The model under review builds one solid part; all positions refer to its coordinate system, in mm. A direction names the side the tool comes from. Give positions to 0.01 mm unless a question says otherwise; leave off trailing zeros. Order: outer loops, then holes, each group sorted by start corner. A loop starts at its lowest first (then second) coordinate and runs counter-clockwise, first axis right, second up. Notation, with made-up numbers: (65.5, -12.5) -> (116.5, -12.5) arc R15 ccw to (116.5, -3.5) -> close; hole circle Ø4 at (32, -22.5). An arc over 180 degrees is marked (long way). Use one line per item in the form item = value.
```python
from build123d import *

# Parameters (mm, degrees)
SKETCH_1_W                   = 310
SKETCH_1_H                   = 120
EXTRUDE_1_DEPTH              = 15
SKETCH_2_W                   = 260
SKETCH_2_H                   = 60
CUT_EXTRUDE_1_DEPTH          = 333.753662639
HOLE_WIZARD_M5_1_D           = 5.8
HOLE_WIZARD_M5_1_CBORE_D     = 10
HOLE_WIZARD_M5_1_CBORE_DEPTH = 5
SKETCH_7_R                   = 3.5
CUT_EXTRUDE_2_DEPTH          = 287.749019179
CHAMFER_1_SIZE               = 10
FILLET_1_R                   = 10
HOLE_WIZARD_M5_1_2_D         = 4.2
HOLE_WIZARD_M5_1_2_DEPTH     = 12.4
HOLE_WIZARD_M5_1_2_TIP       = 1.2618073
SKETCH_10_W                  = 20
SKETCH_10_H                  = 25
CUT_EXTRUDE_3_DEPTH          = 333.753662639


with BuildPart() as part:
    # 草图1 → 凸台-拉伸1 (new body)
    with BuildSketch(Plane.XY):
        with Locations((155, 60)):
            Rectangle(SKETCH_1_W, SKETCH_1_H)
    extrude(amount=EXTRUDE_1_DEPTH)

    # 草图2 → 切除-拉伸1 (cut, through all)
    with BuildSketch(Plane.XY.offset(15)):
        with Locations((180, 90)):
            Rectangle(SKETCH_2_W, SKETCH_2_H)
    extrude(amount=-CUT_EXTRUDE_1_DEPTH, mode=Mode.SUBTRACT)

    # Hole Wizard M5 _1 (through all)
    with Locations(Plane(origin=(0, 60, 0), x_dir=(-1, 0, 0), z_dir=(0, 1, 0))):
        with Locations((-80, 7.5), (-280, 7.5), (-180, 7.5)):
            CounterBoreHole(HOLE_WIZARD_M5_1_D / 2, HOLE_WIZARD_M5_1_CBORE_D / 2, HOLE_WIZARD_M5_1_CBORE_DEPTH)

    # 草图7 → 切除-拉伸2 (cut, through all)
    with BuildSketch(Plane(origin=(50, 0, 0), x_dir=(0, 0, -1), z_dir=(1, 0, 0))):
        with Locations((-7.5, 80)):
            Circle(SKETCH_7_R)
        with Locations((-7.5, 105)):
            Circle(SKETCH_7_R)
    extrude(amount=-CUT_EXTRUDE_2_DEPTH, mode=Mode.SUBTRACT)

    # 倒角1
    chamfer_1_edges = [part.edges().sort_by_distance(p)[0] for p in [
        (310, 60, 7.5),
    ]]
    chamfer(chamfer_1_edges, length=CHAMFER_1_SIZE)

    # 圆角1
    fillet_1_edges = [part.edges().sort_by_distance(p)[0] for p in [
        (50, 60, 7.5),
    ]]
    fillet(fillet_1_edges, radius=FILLET_1_R)

    # Hole Wizard M5 _1 2
    with Locations(Plane(origin=(310, 0, 0), x_dir=(0, 0, -1), z_dir=(1, 0, 0))):
        with Locations((-7.5, 41), (-7.5, 15)):
            Hole(HOLE_WIZARD_M5_1_2_D / 2, depth=HOLE_WIZARD_M5_1_2_DEPTH)
            with Locations((0, 0, -(HOLE_WIZARD_M5_1_2_DEPTH + HOLE_WIZARD_M5_1_2_TIP / 2))):  # 118° drill point
                Cone(0, HOLE_WIZARD_M5_1_2_D / 2, HOLE_WIZARD_M5_1_2_TIP, mode=Mode.SUBTRACT)

    # 草图10 → 切除-拉伸3 (cut, through all)
    with BuildSketch(Plane.XY.offset(15)):
        with Locations((250, 12.5)):
            Rectangle(SKETCH_10_W, SKETCH_10_H)
    extrude(amount=-CUT_EXTRUDE_3_DEPTH, mode=Mode.SUBTRACT)


solid = part.part
```
1. Tool access review of faces 1 (the face through (275.23, 57.54, 9)), 2 (the face through (178.3, 60, 2.6)), 3 (the face through (260, 12, 8)): name each direction out of +Z, -Z, +X, -X, +Y, -Y from which nothing blocks a thin tool from reaching the whole face with its end or side.
Values:
face_1 = +Y
face_2 = +Z, -Z, +X, +Y
face_3 = +Z, -Z, -Y
2. Add section A-A on y = 9. Give the boundary of the cut face in (x, z), then the cut area to 3 significant figures.
Values:
outline = (0, 0) -> (240, 0) -> (240, 15) -> (0, 15) -> close; (260, 0) -> (310, 0) -> (310, 15) -> (260, 15) -> close; hole circle Ø5.8 at (80, 7.5); hole circle Ø5.8 at (180, 7.5); hole circle Ø5.8 at (280, 7.5)
area = 4,270 mm^2
3. Add section D-D on x = 117. Give the boundary of the cut face in (y, z).
Values:
outline = (0, 0) -> (60, 0) -> (60, 15) -> (0, 15) -> close
4. For pin 1 Ø3 at (x, z) = (80.5, 9.5) entering from +Y; pin 2 Ø7.5 at (x, z) = (182, 6.5) entering from +Y, all flat-tipped, find the tip position at first contact; note any pin that passes through.
Values:
pin_1 = 55
pin_2 = 60
5. The part is to be moulded in two halves that separate along Y. For faces 4 (the face through (118, 48, 0)), 5 (the face through (25.35, 76.583, 8.259)), 6 (the face through (285, 0, 7)), say which applies: +Y half, -Y half, draft (parallel to the pull), parting line (faces both ways), or undercut.
Values:
face_4 = draft
face_5 = undercut
face_6 = -Y half
6. For L1, parallel to Y at x = 20, z = 7.5; L2, parallel to Z at x = 304.75, y = 15; L3, parallel to Z at x = 80, y = 56.3, list the stretches that pass through material, from the lowest coordinate up.
Values:
L1 = 0 to 76.5, 83.5 to 101.5, 108.5 to 120
L2 = 0 to 5.4, 9.6 to 15
L3 = 0 to 2.5, 12.5 to 15
7. Add section C-C on y = 105. Give the boundary of the cut face in (x, z), then the cut area to 3 significant figures.
Values:
outline = (0, 0) -> (50, 0) -> (50, 4) -> (0, 4) -> close; (0, 11) -> (50, 11) -> (50, 15) -> (0, 15) -> close
area = 400 mm^2
8. Add section B-B on x = 80. Give the boundary of the cut face in (y, z), then the cut area to 3 significant figures.
Values:
outline = (0, 0) -> (60, 0) -> (60, 2.5) -> (55, 2.5) -> (55, 4.6) -> (0, 4.6) -> close; (0, 10.4) -> (55, 10.4) -> (55, 12.5) -> (60, 12.5) -> (60, 15) -> (0, 15) -> close
area = 531 mm^2
